```python
from build123d import *

# Parameters (mm, degrees)
SKETCH1_R           = 10
BOSS_EXTRUDE1_DEPTH = 32.5
SKETCH2_W           = 6
SKETCH2_H           = 112
BOSS_EXTRUDE2_DEPTH = 10


with BuildPart() as part:
    # Sketch1 → Boss-Extrude1 (new, symmetric)
    with BuildSketch(Plane.YZ):
        with BuildLine():
            Line((-25, 0), (-25, -10))
            ThreePointArc((-25, -10), (-26.464466094, -13.535533906), (-30, -15))
            Line((-30, -15), (-39, -15))
            ThreePointArc((-39, -15), (-42.535533906, -13.535533906), (-44, -10))
            Line((-44, -10), (-44, 0))
            Line((-44, 0), (-56, 0))
            Line((-56, 0), (-56, -25))
            Line((-56, -25), (56, -25))
            Line((56, -25), (56, 0))
            Line((56, 0), (44, 0))
            Line((44, 0), (44, -10))
            ThreePointArc((44, -10), (42.535533906, -13.535533906), (39, -15))
            Line((39, -15), (30, -15))
            ThreePointArc((30, -15), (26.464466094, -13.535533906), (25, -10))
            Line((25, -10), (25, 0))
            ThreePointArc((25, 0), (0, 25), (-25, 0))
        make_face()
        with Locations(Location((0, 0, 0), (0, 0, 270))):
            Circle(SKETCH1_R, mode=Mode.SUBTRACT)
    extrude(amount=BOSS_EXTRUDE1_DEPTH, both=True)

    # Sketch2 → Boss-Extrude2 (add)
    with BuildSketch(Plane(origin=(0, 0, -25), x_dir=(1, 0, 0), z_dir=(0, 0, -1))):
        with Locations((-20, 0)):
            Rectangle(SKETCH2_W, SKETCH2_H)
        with Locations((20, 0)):
            Rectangle(SKETCH2_W, SKETCH2_H)
    extrude(amount=BOSS_EXTRUDE2_DEPTH)


solid = part.part
```
Source: CAD feature listing. Evaluate the final solid. Frame: model axes, mm. A direction names the side the tool comes from. Give positions to 0.01 mm unless a question says otherwise; leave off trailing zeros. Order: outer loops, then holes, each group sorted by start corner. A loop starts at its lowest first (then second) coordinate and runs counter-clockwise, first axis right, second up. Notation, with made-up numbers: (32.5, 43) -> (39.5, 43) arc R27 ccw to (39.5, 66) -> close; hole circle Ø9 at (5, -7.75). An arc over 180 degrees is marked (long way). Use a Markdown table: item, result.
Q1. Section A-A (y = 0). Return the cut outline in (x, z), and give its area (3 significant figures).
A:
| item | result |
|---|---|
| outline | (-32.5, -25) -> (-23, -25) -> (-23, -35) -> (-17, -35) -> (-17, -25) -> (17, -25) -> (17, -35) -> (23, -35) -> (23, -25) -> (32.5, -25) -> (32.5, -10) -> (-32.5, -10) -> close; (-32.5, 10) -> (32.5, 10) -> (32.5, 25) -> (-32.5, 25) -> close |
| area | 2,070 mm^2 |
Q2. Section C-C (y = -15.5). Return the cut outline in (x, z).
A:
| item | result |
|---|---|
| outline | (-32.5, -25) -> (-23, -25) -> (-23, -35) -> (-17, -35) -> (-17, -25) -> (17, -25) -> (17, -35) -> (23, -35) -> (23, -25) -> (32.5, -25) -> (32.5, 19.62) -> (-32.5, 19.62) -> close |
Q3. Pull-direction query (X, two-part tool) for faces 4 (the face through (-32.5, -1, -11)), 5 (the face through (0, 56, -14)), 6 (the face through (-17, 1, -30)); classes: +X half, -X half, draft (parallel to the pull), parting line (faces both ways), or undercut.
A:
| item | result |
|---|---|
| face 4 | -X half |
| face 5 | draft |
| face 6 | undercut |
Q4. Section B-B (x = 10). Return the cut outline in (y, z).
A:
| item | result |
|---|---|
| outline | (-56, -25) -> (56, -25) -> (56, 0) -> (44, 0) -> (44, -10) arc R5 cw to (39, -15) -> (30, -15) arc R5 cw to (25, -10) -> (25, 0) arc R25 ccw to (-25, 0) -> (-25, -10) arc R5 cw to (-30, -15) -> (-39, -15) arc R5 cw to (-44, -10) -> (-44, 0) -> (-56, 0) -> close; hole circle Ø20 at (0, 0) |
Q5. Material intervals for line 1 (X direction, y = -34, z = -29); line 2 (Y direction, x = -7, z = -13.5); line 3 (Z direction, x = 7, y = -46), sorted ascending. Write a range as [from, to].
A:
| item | result |
|---|---|
| line 1 | [-23, -17], [17, 23] |
| line 2 | [-56, -42.57], [-26.43, 26.43], [42.57, 56] |
| line 3 | [-25, 0] |
Q6. Access query for faces 1 (the face through (23, 1, -30)), 2 (the face through (0, 43, -13)), 3 (the face through (0, 50, 0)). Directions: +Z, -Z, +X, -X, +Y, -Y. A direction counts if a zero-diameter tool reaches every point of the face in a straight line with its end or side. Return the directions, or none.
A:
| item | result |
|---|---|
| face 1 | -Z, +X, +Y, -Y |
| face 2 | +Z, +X, -X |
| face 3 | +Z, +X, -X, +Y |
Q7. First-contact query: P1, Ø7, axis at x = 8, y = 35.5, coming from the +Z side; P2, Ø11, axis at y = 6, z = -31, coming from the +X side; P3, Ø3.5, axis at x = -9.5, y = 50, coming from the +Z side. Flat tips, straight axial feed; report the tip coordinate or a pass-through.
A:
| item | result |
|---|---|
| P1 | z = -15 |
| P2 | x = 23 |
| P3 | z = 0 |
